Verification items for this drawing (mm, ordinates from the low corner). A direction names the side the tool comes from. Give positions to 0.01 mm unless a question says otherwise; leave off trailing zeros. Loops run counter-clockwise (first coordinate to the right, second up) from the corner with the lowest first, then second, coordinate; pieces in that order, holes last. Notation, with made-up numbers: (58, 59.25) -> (99, 59.25) arc R30 cw to (99, 95.25) -> close; hole circle Ø8 at (-35.75, 9.5). An arc over 180 degrees is marked (long way). Answer as a JSON object with one key per item and string values.
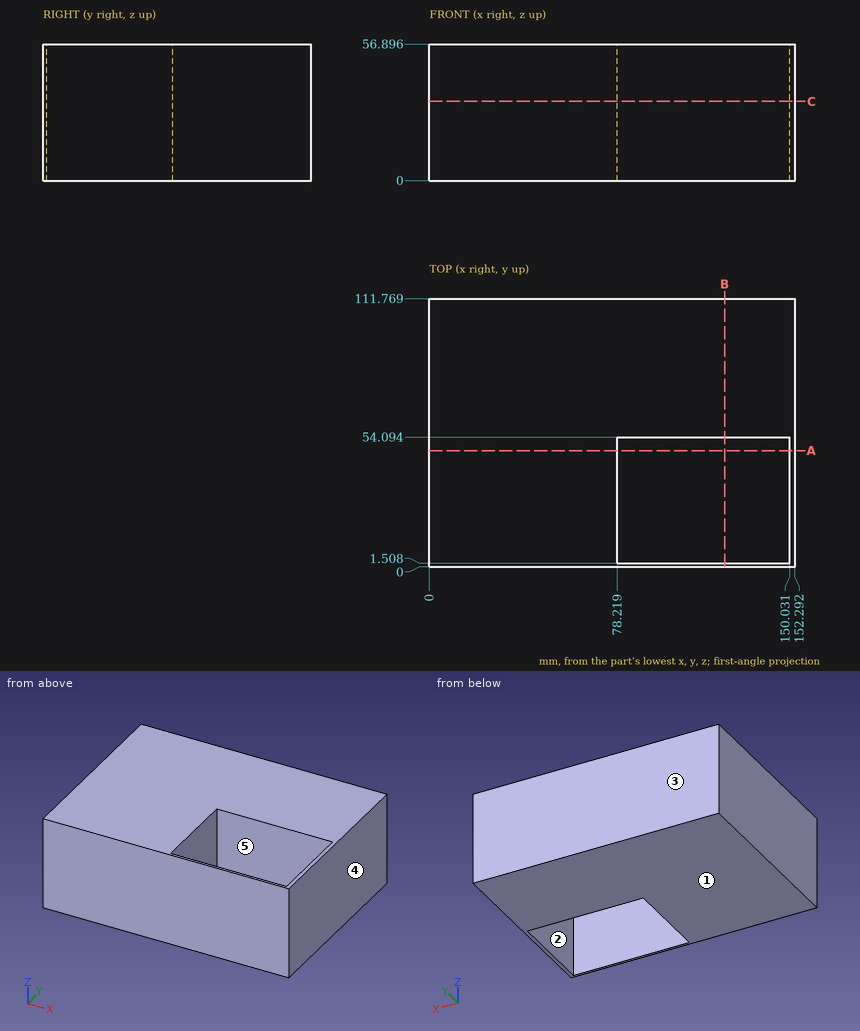
1) Material ranges on line 1 along X through (y, z) = (11, 24.5); line 2 along Y through (x, z) = (114, 27.5), recorded low to high. Write a range as from..to.
Geometry check:
{"line 1": "x = 0..78.22, 150.03..152.29", "line 2": "y = 0..1.51, 54.09..111.77"}
2) Section check B-B on x = 123. Record the cut outline in (y, z).
Geometry check:
{"outline": "(0, 0) -> (1.51, 0) -> (1.51, 56.9) -> (0, 56.9) -> close; (54.09, 0) -> (111.77, 0) -> (111.77, 56.9) -> (54.09, 56.9) -> close"}
3) Section check A-A on y = 48.5. Record the cut outline in (x, z).
Geometry check:
{"outline": "(0, 0) -> (78.22, 0) -> (78.22, 56.9) -> (0, 56.9) -> close; (150.03, 0) -> (152.29, 0) -> (152.29, 56.9) -> (150.03, 56.9) -> close"}
4) Tool access check on the marked faces 1 and 2. Record the directions out of +Z, -Z, +X, -X, +Y, -Y that give a thin tool (end or side, any length) a straight path to the whole face; none if there is none.
Geometry check:
{"face 1": "-Z, +X, -X, +Y, -Y", "face 2": "+Z, -Z"}
5) Section check C-C on z = 33. Record the cut outline in (x, y), plus the area to 3 significant figures.
Geometry check:
{"outline": "(0, 0) -> (152.29, 0) -> (152.29, 111.77) -> (0, 111.77) -> close; hole (78.22, 1.51) -> (150.03, 1.51) -> (150.03, 54.09) -> (78.22, 54.09) -> close", "area": "13,200 mm2"}
6) Draft check along X on the marked faces 3, 4 and 5. Enter one of: pulls with the +X half, pulls with the -X half, needs draft (parallel to the pull), parting line crosses it, or undercut.
Geometry check:
{"face 3": "needs draft", "face 4": "pulls with the +X half", "face 5": "undercut"}
